from build123d import *

# Parameters (mm, degrees)
BOSS_EXTRUDE1_DEPTH = 12
BOSS_EXTRUDE2_DEPTH = 2
BOSS_EXTRUDE3_DEPTH = 3
SKETCH4_W           = 10
SKETCH4_H           = 2
CUT_EXTRUDE1_DEPTH  = 6
SKETCH5_W           = 10
SKETCH5_H           = 2
CUT_EXTRUDE2_DEPTH  = 6
SKETCH6_W           = 10
SKETCH6_H           = 2
CUT_EXTRUDE3_DEPTH  = 6


with BuildPart() as part:
    # Sketch1 → Boss-Extrude1 (new body)
    with BuildSketch(Plane(origin=(0, 0, 0), x_dir=(1, 0, 0), z_dir=(0, 1, 0))):
        Polygon((109.556624327, -4.42820323), (-109.556624327, -4.42820323), (-112.113248654, 0), (-2.55662435, 189.757639654), (2.556624303, 189.757639654), (112.113248654, 0), align=None)
        Polygon((-107.82457352, -1.42820323), (-108.649147039, 0), (-99.473720558, 15.892304845), (-89.473720559, -1.42820323), align=None, mode=Mode.SUBTRACT)
        Polygon((-0.824573543, 186.757639627), (0.824573481, 186.757639627), (9.999999979, 170.86533478), (-10.000000021, 170.86533478), align=None, mode=Mode.SUBTRACT)
        Polygon((108.649147039, 0), (107.824573535, -1.428203221), (89.473720574, -1.428203221), (99.473720574, 15.892304855), align=None, mode=Mode.SUBTRACT)
        Polygon((-11.732050809, 167.865334805), (11.732050809, 167.865334805), (97.741669771, 18.892304864), (86.009618954, -1.428203229), (-86.009618944, -1.428203229), (-97.741669751, 18.892304845), align=None, mode=Mode.SUBTRACT)
    extrude(amount=BOSS_EXTRUDE1_DEPTH)

    # Sketch1<4> → Boss-Extrude2 (add)
    with BuildSketch(Plane(origin=(0, 0, 0), x_dir=(1, 0, 0), z_dir=(0, 1, 0))):
        Polygon((11.732050809, 167.865334805), (-11.732050809, 167.865334805), (-97.741669751, 18.892304845), (-86.009618944, -1.428203229), (86.009618954, -1.428203229), (97.741669771, 18.892304864), align=None)
        with BuildLine():
            Line((-85.566243251, 2.803847594), (-93.854918378, 17.160254041))
            ThreePointArc((-93.854918378, 17.160254041), (-82.532377591, 14.126388381), (-85.566243251, 2.803847594))
        make_face(mode=Mode.SUBTRACT)
        Polygon((-1e-08, 9.732050841), (4.99999999, 1.071796803), (-5.00000001, 1.071796803), align=None, mode=Mode.SUBTRACT)
        Polygon((-45.071796745, 87.798692801), (-55.071796745, 87.798692801), (-50.071796745, 96.458946839), align=None, mode=Mode.SUBTRACT)
        with BuildLine():
            Line((56.226497316, 85.798692796), (94.854918412, 18.892304841))
            Line((94.854918412, 18.892304841), (84.566243293, 1.071796793))
            Line((84.566243293, 1.071796793), (7.309401088, 1.071796793))
            Line((7.309401088, 1.071796793), (2e-09, 13.732050847))
            Line((2e-09, 13.732050847), (-7.309401077, 1.071796786))
            Line((-7.309401077, 1.071796786), (-84.566243251, 1.071796786))
            ThreePointArc((-84.566243251, 1.071796786), (-80.800326783, 15.126388381), (-94.854918378, 18.892304849))
            Line((-94.854918378, 18.892304849), (-56.226497283, 85.798692801))
            Line((-56.226497283, 85.798692801), (-41.60769513, 85.798692801))
            Line((-41.60769513, 85.798692801), (-48.917096207, 98.458946839))
            Line((-48.917096207, 98.458946839), (-10.288675112, 165.365334792))
            Line((-10.288675112, 165.365334792), (-7.309401077, 165.365334792))
            Line((-7.309401077, 165.365334792), (0, 152.705080754))
            Line((0, 152.705080754), (7.309401077, 165.365334792))
            Line((7.309401077, 165.365334792), (10.288675142, 165.365334792))
            Line((10.288675142, 165.365334792), (48.91709624, 98.458946834))
            Line((48.91709624, 98.458946834), (41.607695163, 85.798692796))
            Line((41.607695163, 85.798692796), (56.226497316, 85.798692796))
        make_face(mode=Mode.SUBTRACT)
        Polygon((45.071796778, 87.798692803), (50.071796778, 96.458946841), (55.071796778, 87.798692803), align=None, mode=Mode.SUBTRACT)
        Polygon((0, 156.705080761), (-5, 165.365334799), (5, 165.365334799), align=None, mode=Mode.SUBTRACT)
    extrude(amount=BOSS_EXTRUDE2_DEPTH)

    # Sketch2 → Boss-Extrude3 (add)
    with BuildSketch(Plane.XZ):
        Polygon((101.205771363, -18.892304847), (87.741669751, 4.42820323), (-87.741669751, 4.42820323), (-101.205771368, -18.892304847), (-13.464101652, -170.86533478), (13.464101609, -170.86533478), align=None)
        Polygon((-11.732050819, -167.865334802), (11.732050795, -167.865334802), (97.741669739, -18.892304852), (86.009618931, 1.42820323), (-86.009618931, 1.42820323), (-97.741669763, -18.892304852), align=None, mode=Mode.SUBTRACT)
    extrude(amount=BOSS_EXTRUDE3_DEPTH)

    # Sketch4 → Cut-Extrude1 (cut)
    with BuildSketch(Plane.XY.offset(4.42820323)):
        with Locations((-79.741669751, -1)):
            Rectangle(SKETCH4_W, SKETCH4_H)
    extrude(amount=-CUT_EXTRUDE1_DEPTH, mode=Mode.SUBTRACT)

    # Sketch5 → Cut-Extrude2 (cut)
    with BuildSketch(Plane(origin=(-84.084936503, 0, -48.546460711), x_dir=(-0.4999999998935114, 0, 0.86602540384592), z_dir=(-0.86602540384592, 0, -0.4999999998935114))):
        with Locations((26.241669739, -1)):
            Rectangle(SKETCH5_W, SKETCH5_H)
    extrude(amount=-CUT_EXTRUDE2_DEPTH, mode=Mode.SUBTRACT)

    # Sketch6 → Cut-Extrude3 (cut)
    with BuildSketch(Plane(origin=(84.084936484, 0, -48.546460721), x_dir=(-0.5000000000540236, 0, -0.8660254037532481), z_dir=(0.8660254037532481, 0, -0.5000000000540236))):
        with Locations((53.499999991, -1)):
            Rectangle(SKETCH6_W, SKETCH6_H)
    extrude(amount=-CUT_EXTRUDE3_DEPTH, mode=Mode.SUBTRACT)


solid = part.part
Design review of the part built by this model. Coordinates are the model's own, in mm. A direction names the side the tool comes from. Round coordinates to 2 decimals unless told otherwise and drop trailing zeros. Loops run counter-clockwise (first coordinate to the right, second up) from the corner with the lowest first, then second, coordinate; pieces in that order, holes last. Notation, with made-up numbers: (-37, 47.5) - (3, 47.5) arc R23 ccw to (3, 68.5) - close; hole circle Ø5 at (-23.75, 69). An arc over 180 degrees is marked (long way). One line per item, written item: value. Start each with the question number.
1) To check wall thickness, follow L1, parallel to X at y = 4.5, z = -3.5; L2, parallel to X at y = 10.75, z = -149; L3, parallel to Z at x = -85, y = 1.5. State the ranges of each line that lie inside material, in increasing order. Write a range as from..to.
2) Draft analysis for pull direction X (two halves, no side actions). For faces 4 (the flat face through (-58, 2, -84)), 5 (the flat face through (56.568, 4.605, -96.207)), 6 (the flat face through (107.1, 0, -3)), state which applies: +X half, -X half, draft (parallel to the pull), parting line (faces both ways), or undercut.
3) Insertion check: pin 1 Ø3 at (y, z) = (9, -114) entering from +X; pin 2 Ø3 at (x, y) = (-25.5, 8) entering from -Z; pin 3 Ø6 at (x, y) = (-102, 7.5) entering from -Z. Each pin has a flat end and moves straight along its axis. Give the tip position at first contact, or say it passes through.
4) Consider section B-B on x = 78.5. Give the boundary of the cut face in (y, z).
5) For faces 1 (the flat face through (-55.339, 6.93, -92.336)), 2 (the flat face through (-3.6, 1, -7.5)), 3 (the flat face through (91.958, -1.479, -8.874)), list the 3-axis set-ups (+Z, -Z, +X, -X, +Y, -Y) from which the entire face can be reached by the end or side of a thin tool; tool diameter is ignored.
6) Consider section A-A on y = 7. Give the boundary of the cut face in (x, z).
7) Consider section C-C on z = -42. Give the boundary of the cut face in (x, y), then the cut area to 3 significant figures.
Reported:
1. L1: x = -110.09..-106.63, -92.32..-88.85, 88.85..92.32, 106.63..110.09
1. L2: x = -26.09..-22.62, 22.62..26.09
1. L3: z = -46.96..-35.96, -19.13..-16.8, -3.16..4.43
2. face 4: undercut
2. face 5: +X half
2. face 6: draft
3. pin 1: stops at x = 47.16
3. pin 2: stops at z = -152.62
3. pin 3: stops at z = -22.71
4. outline: (-3, -58.22) - (12, -58.22) - (12, -52.22) - (2, -52.22) - (2, -47.22) - (0, -47.22) - (0, -52.22) - (-3, -52.22) - close; (-3, 1.43) - (0, 1.43) - (0, -1.07) - (2, -1.07) - (2, 1.43) - (12, 1.43) - (12, 4.43) - (-3, 4.43) - close
5. face 1: +Y
5. face 2: +Y, -Y
5. face 3: -Y
6. outline: (-112.11, 0) - (-2.56, -189.76) - (2.56, -189.76) - (112.11, 0) - (109.56, 4.43) - (-109.56, 4.43) - close; hole (-108.65, 0) - (-99.47, -15.89) - (-89.47, 1.43) - (-107.82, 1.43) - close; hole (-97.74, -18.89) - (-11.73, -167.87) - (11.73, -167.87) - (97.74, -18.89) - (86.01, 1.43) - (-86.01, 1.43) - close; hole (-10, -170.87) - (-0.82, -186.76) - (0.82, -186.76) - (10, -170.87) - close; hole (89.47, 1.43) - (99.47, -15.89) - (108.65, 0) - (107.82, 1.43) - close
7. outline: (-87.86, -3) - (-84.4, -3) - (-84.4, 0) - (-81.51, 0) - (-81.51, 2) - (-84.4, 2) - (-84.4, 12) - (-87.86, 12) - close; (81.51, 0) - (84.4, 0) - (84.4, -3) - (87.86, -3) - (87.86, 12) - (84.4, 12) - (84.4, 2) - (81.51, 2) - close
7. area: 115 mm^2
